```python
from build123d import *

# Parameters (mm, degrees)
SKETCH1_W           = 116.62
SKETCH1_H           = 9
BOSS_EXTRUDE1_DEPTH = 2
SKETCH6_R           = 1.5
CUT_EXTRUDE1_DEPTH  = 60.034363721
CHAMFER4_SIZE       = 3
SKETCH9_R           = 1.5
BOSS_EXTRUDE4_DEPTH = 2
BOSS_EXTRUDE5_START = -2
BOSS_EXTRUDE5_DEPTH = 59.2


with BuildPart() as part:
    # Sketch1 → Boss-Extrude1 (new body)
    with BuildSketch(Plane(origin=(0, 0, 0), x_dir=(0, 0, -1), z_dir=(1, 0, 0))):
        with Locations((0, -4.5)):
            Rectangle(SKETCH1_W, SKETCH1_H)
    extrude(amount=BOSS_EXTRUDE1_DEPTH)

    # Sketch6 → Cut-Extrude1 (cut, through all)
    with BuildSketch(Plane.ZY):
        with Locations((0, -4.5)):
            Circle(SKETCH6_R)
        with Locations((52.5, -4.5)):
            Circle(SKETCH6_R)
        with Locations((-52.5, -4.5)):
            Circle(SKETCH6_R)
    extrude(amount=-CUT_EXTRUDE1_DEPTH, mode=Mode.SUBTRACT)

    # Chamfer4
    chamfer4_edges = [part.edges().sort_by_distance(p)[0] for p in [
        (1, -9, -58.31),
        (1, -9, 58.31),
    ]]
    chamfer(chamfer4_edges, length=CHAMFER4_SIZE)



with BuildPart() as body_2:
    # Sketch9 → Boss-Extrude4 (new body)
    with BuildSketch(Plane(origin=(57.2, 0, 0), x_dir=(0, 0, -1), z_dir=(1, 0, 0))):
        Polygon((-58.31, 0), (-58.31, -6), (-55.31, -9), (55.31, -9), (58.31, -6), (58.31, 0), align=None)
        with Locations(Location((0, -4.5, 0), (0, 0, 180))):
            Circle(SKETCH9_R, mode=Mode.SUBTRACT)
        with Locations(Location((-52.5, -4.5, 0), (0, 0, 180))):
            Circle(SKETCH9_R, mode=Mode.SUBTRACT)
        with Locations(Location((52.5, -4.5, 0), (0, 0, 180))):
            Circle(SKETCH9_R, mode=Mode.SUBTRACT)
    extrude(amount=BOSS_EXTRUDE4_DEPTH)


with BuildPart() as part_1:
    add(part.part)

    add(body_2.part)  # Boss-Extrude5 merges body 2
    # Sketch4 → Boss-Extrude5 (add)
    with BuildSketch(Plane(origin=(2, 0, 0), x_dir=(0, 0, -1), z_dir=(1, 0, 0)).offset(BOSS_EXTRUDE5_START)):
        Polygon((-58.31, 0), (-51.811665078, 3), (52.525651767, 3), (58.31, 0), align=None)
    extrude(amount=BOSS_EXTRUDE5_DEPTH)


solid = part_1.part
```
Here's how the part is built. I have some questions about the finished solid (model axes, mm). A direction names the side the tool comes from. Coordinates: 2 decimals unless noted, no trailing zeros. Loops run counter-clockwise (first coordinate to the right, second up) from the corner with the lowest first, then second, coordinate; pieces in that order, holes last. Notation, with made-up numbers: (61, 87) - (115, 87) arc R19 cw to (115, 106) - close; hole circle Ø1 at (28, 36). An arc over 180 degrees is marked (long way). Answer as CSV lines item,"result".
Q1. We'd pull the mould along X, two halves only. Please class faces 3 (the face through (57.2, -6, 1)), 4 (the face through (58.2, -3.6, 51.3)), 5 (the face through (0, -3, -1)), 6 (the face through (59.2, -3, -1)): pulls with the +X half, pulls with the -X half, needs draft (parallel to the pull), parting line crosses it, or undercut.
Response:
face 3,"undercut"
face 4,"needs draft"
face 5,"pulls with the -X half"
face 6,"pulls with the +X half"
Q2. If we section it at C-C, the plane z = -38: Write out the boundary of the cut face in (x, y).
Response:
outline,"(0, -9) - (2, -9) - (2, 0) - (57.2, 0) - (57.2, -9) - (59.2, -9) - (59.2, 3) - (0, 3) - close"
Q3. For faces 1 (the face through (29, 0, -1)), 2 (the face through (58.19, -7.52, -56.79)), which set-ups out of +Z, -Z, +X, -X, +Y, -Y let a thin tool reach every point of the face, with its end or its side?
Response:
face 1,"+Z, -Z, -Y"
face 2,"-Z, +X, -X, -Y"
Q4. For pin 1 (1.5 mm diameter, centred on x = 25, y = -1.5, fed in from -Z); pin 2 (2 mm diameter, centred on x = 11, z = 11.5, fed in from -Y), each with a flat end and sliding along its axis, tell me the tip position at first contact or that it passes through.
Response:
pin 1,"through"
pin 2,"y = 0"
Q5. If I drill on L1, parallel to Y at x = 58.65, z = -52.5; L2, parallel to X at y = -1.75, z = -24; L3, parallel to Y at x = 26.5, z = -40, over which ranges is the centre line in solid material (lowest first)? Write a range as [from, to].
Response:
L1,"[-9, -6], [-3, 3]"
L2,"[0, 2], [57.2, 59.2]"
L3,"[0, 3]"
Q6. If we section it at A-A, the plane z = 0: Write out the boundary of the cut face in (x, y), and give its area (3 significant figures).
Response:
outline,"(0, -9) - (2, -9) - (2, -6) - (0, -6) - close; (0, -3) - (2, -3) - (2, 0) - (57.2, 0) - (57.2, -3) - (59.2, -3) - (59.2, 3) - (0, 3) - close; (57.2, -9) - (59.2, -9) - (59.2, -6) - (57.2, -6) - close"
area,"202 mm2"
Q7. If we section it at B-B, the plane y = -4.5: Give the number of separate pieces and of enclosed holes in the cut face, and give its area (3 significant figures).
Response:
separate pieces,"8"
enclosed holes,"0"
area,"430 mm2"
Q8. If we section it at D-D, the plane x = 55: Write out the boundary of the cut face in (y, z), and give its area (3 significant figures).
Response:
outline,"(0, -58.31) - (3, -52.53) - (3, 51.81) - (0, 58.31) - close"
area,"331 mm2"
